Part model, mm, in its own coordinate system. A direction names the side the tool comes from. Round coordinates to 2 decimals unless told otherwise and drop trailing zeros. Loops run counter-clockwise (first coordinate to the right, second up) from the corner with the lowest first, then second, coordinate; pieces in that order, holes last. Notation, with made-up numbers: (66, -22.5) -> (107, -22.5) arc R15 ccw to (107, -3.5) -> close; hole circle Ø5 at (50.5, 16.25). An arc over 180 degrees is marked (long way). Use a Markdown table: item, result. Add a question column.
Item 1: Cut at C-C, the plane x = -63. List the corners of the cut face in (y, z), plus the area to 3 significant figures.
Item 2: Two-plate mould, pull along X, no slides. Class faces 5 (the face through (-17, 14, 2)), 6 (the face through (-69.14, -9.1, 2.54)): pulls with the +X half, pulls with the -X half, needs draft (parallel to the pull), parting line crosses it, or undercut.
Item 3: Cut at A-A, the plane x = 0.5. List the corners of the cut face in (y, z).
Item 4: Probe line 1 (X direction, y = 73.85, z = 4.3); line 2 (X direction, y = -6, z = 4); line 3 (Y direction, x = -63, z = 4.2). List the from-to ranges inside material, lowest first. Write a range as [from, to].
Item 5: Flat gauge pins, fed straight in: pin 1 (3.5 mm diameter, centred on x = -30, y = -6, fed in from -Z); pin 2 (3.5 mm diameter, centred on x = -63, y = 73.85, fed in from +Z); pin 3 (1.4 mm diameter, centred on x = 42, y = 76, fed in from +Z). Where does each tip first touch, or does it go through?
Item 6: Cut at B-B, the plane y = 39.5. List the corners of the cut face in (x, z).
Item 7: Which spindle directions (+Z, -Z, +X, -X, +Y, -Y) get a long thin tool onto all of the face, cutting with end or side? Do faces 1 (the face through (-65.619, 19.958, 4.113)), 2 (the face through (22.14, 66.1, 2.54)), 3 (the face through (39.6, 74.2, 1.5)), 4 (the face through (-70, 34, 2)). Say none if no direction does.
```python
from build123d import *

# Parameters (mm, degrees)
CYLINDER051_R             = 1
CYLINDER051_DEPTH         = 25
CYLINDER052_R             = 1
CYLINDER052_DEPTH         = 25
CYLINDER053_R             = 1
CYLINDER053_DEPTH         = 25
CYLINDER057_R             = 3
CYLINDER057_DEPTH         = 2
CYLINDER058_R             = 3
CYLINDER058_DEPTH         = 2
CYLINDER059_R             = 3
CYLINDER059_DEPTH         = 2
CYLINDER060_R             = 3
CYLINDER060_DEPTH         = 2
CYLINDER050_R             = 1
CYLINDER050_DEPTH         = 25
CYLINDER020_R             = 3.3
CYLINDER020_DEPTH         = 2
CYLINDER019_R             = 3.3
CYLINDER019_DEPTH         = 2
CYLINDER017_R             = 3.3
CYLINDER017_DEPTH         = 2
CYLINDER018_R             = 3.3
CYLINDER018_DEPTH         = 2
FUSION015_PLACEMENT_ANGLE = 180
CYLINDER016_R             = 1.6
CYLINDER016_DEPTH         = 6
CYLINDER013_R             = 1.6
CYLINDER013_DEPTH         = 6
CYLINDER012_R             = 1.6
CYLINDER012_DEPTH         = 6
CYLINDER015_R             = 1.6
CYLINDER015_DEPTH         = 6
CYLINDER014_R             = 1.2
CYLINDER014_DEPTH         = 4.2
FUSION014_PLACEMENT_ANGLE = 180
CYLINDER030_R             = 1.2
CYLINDER030_DEPTH         = 12
CYLINDER031_R             = 1.2
CYLINDER031_DEPTH         = 12
CYLINDER032_R             = 1.2
CYLINDER032_DEPTH         = 12
CYLINDER033_R             = 1.2
CYLINDER033_DEPTH         = 12
CYLINDER034_R             = 3
CYLINDER034_DEPTH         = 3
CYLINDER035_R             = 3
CYLINDER035_DEPTH         = 3
CYLINDER036_R             = 3
CYLINDER036_DEPTH         = 3
CYLINDER037_R             = 3
CYLINDER037_DEPTH         = 3
BOX039_W                  = 78
BOX039_H                  = 53
BOX039_DEPTH              = 6
FILLET002029_R            = 3
BOX017_W                  = 128
BOX017_H                  = 90
BOX017_DEPTH              = 5
FILLET002014_R            = 3


with BuildPart() as obj1:
    # Cylinder051 → Cylinder051 (new body)
    with BuildSketch(Plane(origin=(-30, 9, 0), x_dir=(1, 0, 0), z_dir=(0, 0, 1))):
        Circle(CYLINDER051_R)
    extrude(amount=CYLINDER051_DEPTH)


with BuildPart() as obj2:
    # Cylinder052 → Cylinder052 (new body)
    with BuildSketch(Plane(origin=(15, -6, 0), x_dir=(1, 0, 0), z_dir=(0, 0, 1))):
        Circle(CYLINDER052_R)
    extrude(amount=CYLINDER052_DEPTH)


with BuildPart() as obj3:
    # Cylinder053 → Cylinder053 (new body)
    with BuildSketch(Plane(origin=(15, 9, 0), x_dir=(1, 0, 0), z_dir=(0, 0, 1))):
        Circle(CYLINDER053_R)
    extrude(amount=CYLINDER053_DEPTH)


with BuildPart() as obj4:
    # Cylinder057 → Cylinder057 (new body)
    with BuildSketch(Plane(origin=(15, -6, 0), x_dir=(1, 0, 0), z_dir=(0, 0, 1))):
        Circle(CYLINDER057_R)
    extrude(amount=CYLINDER057_DEPTH)


with BuildPart() as obj5:
    # Cylinder058 → Cylinder058 (new body)
    with BuildSketch(Plane(origin=(-30, -6, 0), x_dir=(1, 0, 0), z_dir=(0, 0, 1))):
        Circle(CYLINDER058_R)
    extrude(amount=CYLINDER058_DEPTH)


with BuildPart() as obj6:
    # Cylinder059 → Cylinder059 (new body)
    with BuildSketch(Plane(origin=(-30, 9, 0), x_dir=(1, 0, 0), z_dir=(0, 0, 1))):
        Circle(CYLINDER059_R)
    extrude(amount=CYLINDER059_DEPTH)


with BuildPart() as obj7:
    # Cylinder060 → Cylinder060 (new body)
    with BuildSketch(Plane(origin=(15, 9, 0), x_dir=(1, 0, 0), z_dir=(0, 0, 1))):
        Circle(CYLINDER060_R)
    extrude(amount=CYLINDER060_DEPTH)


with BuildPart() as fusion032002:
    # Cylinder050 → Cylinder050 (new body)
    with BuildSketch(Plane(origin=(-30, -6, 0), x_dir=(1, 0, 0), z_dir=(0, 0, 1))):
        Circle(CYLINDER050_R)
    extrude(amount=CYLINDER050_DEPTH)

    # Fusion032002: union obj1, obj2, obj3, obj4, obj5, obj6, obj7
    add(obj1.part)
    add(obj2.part)
    add(obj3.part)
    add(obj4.part)
    add(obj5.part)
    add(obj6.part)
    add(obj7.part)


with BuildPart() as cylinder020:
    # Cylinder020 → Cylinder020 (new body)
    with BuildSketch(Plane(origin=(46.85, -27.85, 2), x_dir=(1, 0, 0), z_dir=(0, 0, 1))):
        Circle(CYLINDER020_R)
    extrude(amount=CYLINDER020_DEPTH)


with BuildPart() as cylinder019:
    # Cylinder019 → Cylinder019 (new body)
    with BuildSketch(Plane(origin=(-47, -27.85, 2), x_dir=(1, 0, 0), z_dir=(0, 0, 1))):
        Circle(CYLINDER019_R)
    extrude(amount=CYLINDER019_DEPTH)


with BuildPart() as cylinder017:
    # Cylinder017 → Cylinder017 (new body)
    with BuildSketch(Plane(origin=(-47, 28.05, 2), x_dir=(1, 0, 0), z_dir=(0, 0, 1))):
        Circle(CYLINDER017_R)
    extrude(amount=CYLINDER017_DEPTH)


with BuildPart() as obj8:
    # Cylinder018 → Cylinder018 (new body)
    with BuildSketch(Plane(origin=(46.85, 28.05, 2), x_dir=(1, 0, 0), z_dir=(0, 0, 1))):
        Circle(CYLINDER018_R)
    extrude(amount=CYLINDER018_DEPTH)

    # Fusion015: union Cylinder020, Cylinder019, Cylinder017
    add(cylinder020.part)
    add(cylinder019.part)
    add(cylinder017.part)


with BuildPart() as obj8_1:
    # Fusion015 placement: moved
    add(obj8.part.moved(Location((-51, 46, 7.2))).rotate(Axis((-51, 46, 7.2), (1, 0, 0)), FUSION015_PLACEMENT_ANGLE))


with BuildPart() as cylinder016:
    # Cylinder016 → Cylinder016 (new body)
    with BuildSketch(Plane(origin=(46.85, 28.05, 1.2), x_dir=(1, 0, 0), z_dir=(0, 0, 1))):
        Circle(CYLINDER016_R)
    extrude(amount=CYLINDER016_DEPTH)


with BuildPart() as cylinder013:
    # Cylinder013 → Cylinder013 (new body)
    with BuildSketch(Plane(origin=(46.85, -27.85, 1.2), x_dir=(1, 0, 0), z_dir=(0, 0, 1))):
        Circle(CYLINDER013_R)
    extrude(amount=CYLINDER013_DEPTH)


with BuildPart() as cylinder012:
    # Cylinder012 → Cylinder012 (new body)
    with BuildSketch(Plane(origin=(-47, -27.85, 1.2), x_dir=(1, 0, 0), z_dir=(0, 0, 1))):
        Circle(CYLINDER012_R)
    extrude(amount=CYLINDER012_DEPTH)


with BuildPart() as cylinder015:
    # Cylinder015 → Cylinder015 (new body)
    with BuildSketch(Plane(origin=(-47, 28.05, 1.2), x_dir=(1, 0, 0), z_dir=(0, 0, 1))):
        Circle(CYLINDER015_R)
    extrude(amount=CYLINDER015_DEPTH)


with BuildPart() as obj9:
    # Cylinder014 → Cylinder014 (new body)
    with BuildSketch(Plane(origin=(46.85, -15.5, -2.3), x_dir=(0, 0, -1), z_dir=(1, 0, 0))):
        Circle(CYLINDER014_R)
    extrude(amount=CYLINDER014_DEPTH)

    # Fusion014: union Cylinder016, Cylinder013, Cylinder012, Cylinder015
    add(cylinder016.part)
    add(cylinder013.part)
    add(cylinder012.part)
    add(cylinder015.part)


with BuildPart() as obj9_1:
    # Fusion014 placement: moved
    add(obj9.part.moved(Location((-51, 46, 7.2))).rotate(Axis((-51, 46, 7.2), (1, 0, 0)), FUSION014_PLACEMENT_ANGLE))

    # Fusion: union obj8
    add(obj8_1.part)


with BuildPart() as obj9_2:
    # Fusion placement: moved
    add(obj9_1.part.moved(Location((35, 0, 0))))


with BuildPart() as obj10:
    # Cylinder030 → Cylinder030 (new body)
    with BuildSketch(Plane(origin=(54, 47, 0), x_dir=(1, 0, 0), z_dir=(0, 0, 1))):
        Circle(CYLINDER030_R)
    extrude(amount=CYLINDER030_DEPTH)


with BuildPart() as obj11:
    # Cylinder031 → Cylinder031 (new body)
    with BuildSketch(Plane(origin=(42, 47, 0), x_dir=(1, 0, 0), z_dir=(0, 0, 1))):
        Circle(CYLINDER031_R)
    extrude(amount=CYLINDER031_DEPTH)


with BuildPart() as obj12:
    # Cylinder032 → Cylinder032 (new body)
    with BuildSketch(Plane(origin=(54, 76, 0), x_dir=(1, 0, 0), z_dir=(0, 0, 1))):
        Circle(CYLINDER032_R)
    extrude(amount=CYLINDER032_DEPTH)


with BuildPart() as obj13:
    # Cylinder033 → Cylinder033 (new body)
    with BuildSketch(Plane(origin=(42, 76, 0), x_dir=(1, 0, 0), z_dir=(0, 0, 1))):
        Circle(CYLINDER033_R)
    extrude(amount=CYLINDER033_DEPTH)


with BuildPart() as obj14:
    # Cylinder034 → Cylinder034 (new body)
    with BuildSketch(Plane(origin=(54, 47, 0), x_dir=(1, 0, 0), z_dir=(0, 0, 1))):
        Circle(CYLINDER034_R)
    extrude(amount=CYLINDER034_DEPTH)


with BuildPart() as obj15:
    # Cylinder035 → Cylinder035 (new body)
    with BuildSketch(Plane(origin=(42, 47, 0), x_dir=(1, 0, 0), z_dir=(0, 0, 1))):
        Circle(CYLINDER035_R)
    extrude(amount=CYLINDER035_DEPTH)


with BuildPart() as obj16:
    # Cylinder036 → Cylinder036 (new body)
    with BuildSketch(Plane(origin=(54, 76, 0), x_dir=(1, 0, 0), z_dir=(0, 0, 1))):
        Circle(CYLINDER036_R)
    extrude(amount=CYLINDER036_DEPTH)


with BuildPart() as obj17:
    # Cylinder037 → Cylinder037 (new body)
    with BuildSketch(Plane(origin=(42, 76, 0), x_dir=(1, 0, 0), z_dir=(0, 0, 1))):
        Circle(CYLINDER037_R)
    extrude(amount=CYLINDER037_DEPTH)

    # Fusion030: union obj10, obj11, obj12, obj13, obj14, obj15, obj16
    add(obj10.part)
    add(obj11.part)
    add(obj12.part)
    add(obj13.part)
    add(obj14.part)
    add(obj15.part)
    add(obj16.part)


with BuildPart() as fusion031:
    # Box039 → Box039 (new body)
    with BuildSketch(Plane(origin=(-55, 14, 0), x_dir=(1, 0, 0), z_dir=(0, 0, 1))):
        with Locations((39, 26.5)):
            Rectangle(BOX039_W, BOX039_H)
    extrude(amount=BOX039_DEPTH)

    # Fillet002029
    fillet002029_edges = [fusion031.edges().sort_by_distance(p)[0] for p in [
        (-55, 14, 3),
        (-55, 67, 3),
        (23, 14, 3),
        (23, 67, 3),
    ]]
    fillet(fillet002029_edges, radius=FILLET002029_R)

    # Fusion031: union obj9, obj17
    add(obj9_2.part)
    add(obj17.part)


with BuildPart() as obj18:
    # Box017 → Box017 (new body)
    with BuildSketch(Plane(origin=(-70, -10, 0), x_dir=(1, 0, 0), z_dir=(0, 0, 1))):
        with Locations((64, 45)):
            Rectangle(BOX017_W, BOX017_H)
    extrude(amount=BOX017_DEPTH)

    # Fillet002014
    fillet002014_edges = [obj18.edges().sort_by_distance(p)[0] for p in [
        (-70, -10, 2.5),
        (-70, 80, 2.5),
        (58, -10, 2.5),
        (58, 80, 2.5),
    ]]
    fillet(fillet002014_edges, radius=FILLET002014_R)

    # Cut: cut Fusion031
    add(fusion031.part, mode=Mode.SUBTRACT)

    # Cut010: cut Fusion032002
    add(fusion032002.part, mode=Mode.SUBTRACT)


solid = obj18.part
```
A:
| question | item | result |
|---|---|---|
| 1 | outline | (-10, 0) -> (16.35, 0) -> (16.35, 3.2) -> (14.65, 3.2) -> (14.65, 5) -> (-10, 5) -> close; (19.55, 0) -> (72.25, 0) -> (72.25, 3.2) -> (70.55, 3.2) -> (70.55, 5) -> (21.25, 5) -> (21.25, 3.2) -> (19.55, 3.2) -> close; (75.45, 0) -> (80, 0) -> (80, 5) -> (77.15, 5) -> (77.15, 3.2) -> (75.45, 3.2) -> close |
| 1 | area | 406 mm^2 |
| 2 | face 5 | undercut |
| 2 | face 6 | pulls with the -X half |
| 3 | outline | (-10, 0) -> (14, 0) -> (14, 5) -> (-10, 5) -> close; (67, 0) -> (80, 0) -> (80, 5) -> (67, 5) -> close |
| 4 | line 1 | x = [-70, -66.3], [-59.7, 27.55], [34.15, 58] |
| 4 | line 2 | x = [-70, -31], [-29, 14], [16, 58] |
| 4 | line 3 | y = [-10, 14.65], [21.25, 70.55], [77.15, 80] |
| 5 | pin 1 | stops at z = 2 |
| 5 | pin 2 | stops at z = 3.2 |
| 5 | pin 3 | passes through |
| 6 | outline | (-70, 0) -> (-55, 0) -> (-55, 5) -> (-70, 5) -> close; (23, 0) -> (58, 0) -> (58, 5) -> (23, 5) -> close |
| 7 | face 1 | +Z |
| 7 | face 2 | +Z, -Z |
| 7 | face 3 | -Z |
| 7 | face 4 | +Z, -Z, -X, +Y, -Y |
